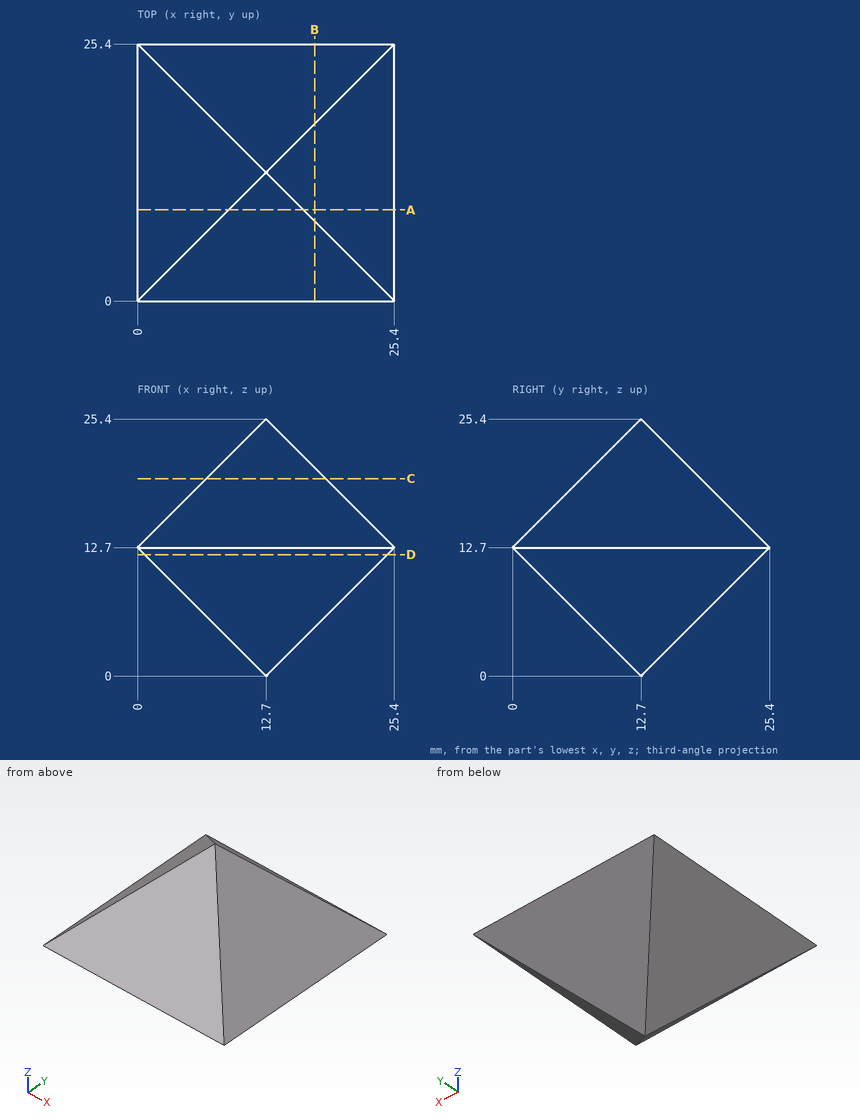
Check sheet for the drawn part. Datum: minimum x, y, z corner. Units: mm. Coordinates: 2 decimals unless noted, no trailing zeros. Order: outer loops, then holes, each group sorted by start corner. A loop starts at its lowest first (then second) coordinate and runs counter-clockwise, first axis right, second up. Notation, with made-up numbers: (-38.5, 48.5) -> (7.5, 48.5) arc R18 cw to (7.5, 78.5) -> close; hole circle Ø5 at (19.5, 5). An arc over 180 degrees is marked (long way). Use a Markdown table: item, result. Add a question column.
1. Cross-section at D-D (z = 12). Enter the section's corners in (x, y).
2. Material ranges on L1, parallel to Z at x = 20, y = 23; L2, parallel to Z at x = 18.75, y = 11.5; L3, parallel to X at y = 10.75, z = 16.75, recorded low to high.
3. Cross-section at A-A (y = 9). Enter the section's corners in (x, z).
4. Cross-section at C-C (z = 19.5). Enter the section's corners in (x, y).
5. Go/stop test with flat-tipped pins: pin 1 Ø3 at (x, y) = (22.5, 20.5) entering from -Z; pin 2 Ø1.5 at (x, z) = (10.5, 8) entering from -Y; pin 3 Ø12 at (x, z) = (2.5, 10) entering from -Y; pin 4 Ø3 at (x, z) = (6.5, 9.5) entering from -Y. Record where each tip stops, or that it passes through.
6. Cross-section at B-B (x = 17.5). Enter the section's corners in (y, z), and give its area (4 significant figures).
Filled sheet:
| question | item | result |
|---|---|---|
| 1 | outline | (0.7, 0.7) -> (24.7, 0.7) -> (24.7, 24.7) -> (0.7, 24.7) -> close |
| 2 | L1 | 10.3 to 15.1 |
| 2 | L2 | 6.05 to 19.35 |
| 2 | L3 | 4.05 to 21.35 |
| 3 | outline | (0, 12.7) -> (9, 3.7) -> (16.4, 3.7) -> (25.4, 12.7) -> (16.4, 21.7) -> (9, 21.7) -> close |
| 4 | outline | (6.8, 6.8) -> (18.6, 6.8) -> (18.6, 18.6) -> (6.8, 18.6) -> close |
| 5 | pin 1 | z = 8.3 |
| 5 | pin 2 | y = 3.95 |
| 5 | pin 3 | y = 0 |
| 5 | pin 4 | y = 1.7 |
| 6 | outline | (0, 12.7) -> (7.9, 4.8) -> (17.5, 4.8) -> (25.4, 12.7) -> (17.5, 20.6) -> (7.9, 20.6) -> close |
| 6 | area | 276.5 mm2 |
